from build123d import *

# Parameters (mm, degrees)
SKETCH1_W           = 70
SKETCH1_H           = 85
BOSS_EXTRUDE1_DEPTH = 5
SKETCH2_R           = 2.1
CUT_EXTRUDE1_DEPTH  = 5
BOSS_EXTRUDE2_DEPTH = 5


with BuildPart() as part:
    # Sketch1 → Boss-Extrude1 (new body)
    with BuildSketch(Plane.XY):
        Rectangle(SKETCH1_W, SKETCH1_H)
    extrude(amount=BOSS_EXTRUDE1_DEPTH)

    # Sketch2 → Cut-Extrude1 (cut)
    with BuildSketch(Plane.XY.offset(5)):
        with Locations((0, -15)):
            Circle(SKETCH2_R)
        with Locations((0, -40)):
            Circle(SKETCH2_R)
        Polygon((2.1, 42.5), (2.1, 37.5), (5, 37.5), (5, 27.5), (-5, 27.5), (-5, 37.5), (-2.1, 37.5), (-2.1, 42.5), align=None)
    extrude(amount=-CUT_EXTRUDE1_DEPTH, mode=Mode.SUBTRACT)

    # Sketch3 → Boss-Extrude2 (add)
    with BuildSketch(Plane.XY.offset(5)):
        with BuildLine():
            Line((-4.330127019, -42.5), (4.330127019, -42.5))
            ThreePointArc((4.330127019, -42.5), (0, -45), (-4.330127019, -42.5))
        make_face()
    extrude(amount=-BOSS_EXTRUDE2_DEPTH)


solid = part.part
CAD build for the part. Positions are in the model's coordinates, mm. A direction names the side the tool comes from. Round coordinates to 2 decimals unless told otherwise and drop trailing zeros. Write each loop counter-clockwise with the first axis right and the second up, starting at its lowest first coordinate (ties: lowest second). Pieces come first, ordered by that corner, then holes.
(1) Slice it at A-A, the plane x = 0. Write the cut outline in (y, z), and give its area (4 significant figures).
(2) Probe line 1 along Y through (x, z) = (0, 1.25); line 2 along X through (y, z) = (38, 4.35); line 3 along Y through (x, z) = (-19, 3.15). List the from-to ranges inside material, lowest first.
(3) Slice it at B-B, the plane y = -15. Write the cut outline in (x, z), and give its area (3 significant figures).
(4) Slice it at C-C, the plane z = 2.7. Write the cut outline in (x, y), and give its area (3 significant figures).
(5) Drop flat-ended pins along their axis: P1, Ø1, axis at x = 18, y = -1, coming from the -Z side; P2, Ø2.5, axis at x = 20.5, z = 2, coming from the -Y side; P3, Ø0.9, axis at x = 3.5, z = 2, coming from the -Y side; P4, Ø3, axis at x = -4, z = 3, coming from the -Y side. Give the stop position or say it passes through.
(6) Mould opens along X. For faces 6 (the face through (-35, -1, 2)), 7 (the face through (-4, 37.5, 3)), 8 (the face through (-20, -42.5, 2)) say: pulls with the +X half, pulls with the -X half, needs draft (parallel to the pull), parting line crosses it, or undercut.
(7) 3-axis set-ups, long thin cutter, end or side, ignore diameter. For faces 1 (the face through (19, -42.5, 2)), 2 (the face through (0, 27.5, 3)), 3 (the face through (0, -1, 0)), 4 (the face through (2.1, 40, 3)), 5 (the face through (0, -1, 5)): which of +Z, -Z, +X, -X, +Y, -Y reach the whole face in a straight line?
(8) Slice it at D-D, the plane x = -29. Write the cut outline in (y, z), and give its area (3 significant figures).
From the geometry:
1. outline: (-45, 0) - (-42.1, 0) - (-42.1, 5) - (-45, 5) - close; (-37.9, 0) - (-17.1, 0) - (-17.1, 5) - (-37.9, 5) - close; (-12.9, 0) - (27.5, 0) - (27.5, 5) - (-12.9, 5) - close
1. area: 320.5 mm2
2. line 1: y = -45 to -42.1, -37.9 to -17.1, -12.9 to 27.5
2. line 2: x = -35 to -2.1, 2.1 to 35
2. line 3: y = -42.5 to 42.5
3. outline: (-35, 0) - (-2.1, 0) - (-2.1, 5) - (-35, 5) - close; (2.1, 0) - (35, 0) - (35, 5) - (2.1, 5) - close
3. area: 329 mm2
4. outline: (-35, -42.5) - (-4.33, -42.5) arc R5 ccw to (4.33, -42.5) - (35, -42.5) - (35, 42.5) - (2.1, 42.5) - (2.1, 37.5) - (5, 37.5) - (5, 27.5) - (-5, 27.5) - (-5, 37.5) - (-2.1, 37.5) - (-2.1, 42.5) - (-35, 42.5) - close; hole circle Ø4.2 at (0, -40); hole circle Ø4.2 at (0, -15)
4. area: 5,820 mm2
5. P1: stops at z = 0
5. P2: stops at y = -42.5
5. P3: stops at y = -43.96
5. P4: stops at y = -44.33
6. face 6: pulls with the -X half
6. face 7: undercut
6. face 8: needs draft
7. face 1: +Z, -Z, +X, -Y
7. face 2: +Z, -Z
7. face 3: -Z, +X, -X, +Y, -Y
7. face 4: +Z, -Z, +Y
7. face 5: +Z, +X, -X, +Y, -Y
8. outline: (-42.5, 0) - (42.5, 0) - (42.5, 5) - (-42.5, 5) - close
8. area: 425 mm2
